from build123d import *

# Parameters (mm, degrees)
SKETCH_1_R             = 2.1
SKETCH_1_R_2           = 1.6
EXTRUDE_1_DEPTH        = 3
HOLE_WIZARD_1_D        = 3.5
HOLE_WIZARD_2_D        = 3.3
PATTERN_LINEAR_1_COUNT = 7
PATTERN_LINEAR_1_PITCH = 15
PATTERN_LINEAR_2_COUNT = 4
PATTERN_LINEAR_2_PITCH = 10
HOLE_WIZARD_3_D        = 3.3
PATTERN_LINEAR_3_COUNT = 7
PATTERN_LINEAR_3_PITCH = 10
HOLE_WIZARD_4_D        = 3.3
SKETCH_14_W            = 20
SKETCH_14_H            = 20
CUT_EXTRUDE_1_DEPTH    = 10
FILLET_1_R             = 3


with BuildPart() as part:
    # 草图1 → 凸台-拉伸1 (new body)
    with BuildSketch(Plane(origin=(0, 0, 0), x_dir=(1, 0, 0), z_dir=(0, 1, 0))):
        with BuildLine():
            Line((-95, 3), (-95, 209))
            ThreePointArc((-95, 209), (-94.121320344, 211.121320344), (-92, 212))
            Line((-92, 212), (92, 212))
            ThreePointArc((92, 212), (94.121320344, 211.121320344), (95, 209))
            Line((95, 209), (95, 3))
            ThreePointArc((95, 3), (94.121320344, 0.878679656), (92, 0))
            Line((92, 0), (56, 0))
            ThreePointArc((56, 0), (53.878679656, 0.878679656), (53, 3))
            Line((53, 3), (53, 43))
            ThreePointArc((53, 43), (44.213203436, 64.213203436), (23, 73))
            Line((23, 73), (-23, 73))
            ThreePointArc((-23, 73), (-44.213203436, 64.213203436), (-53, 43))
            Line((-53, 43), (-53, 3))
            ThreePointArc((-53, 3), (-53.878679656, 0.878679656), (-56, 0))
            Line((-56, 0), (-92, 0))
            ThreePointArc((-92, 0), (-94.121320344, 0.878679656), (-95, 3))
        make_face()
        with Locations(Location((-11.75, 96.75, 0), (0, 0, 270))):
            Circle(SKETCH_1_R, mode=Mode.SUBTRACT)
        with Locations(Location((11.75, 96.75, 0), (0, 0, 270))):
            Circle(SKETCH_1_R, mode=Mode.SUBTRACT)
        with Locations(Location((11.75, 79.25, 0), (0, 0, 270))):
            Circle(SKETCH_1_R, mode=Mode.SUBTRACT)
        with Locations(Location((-11.75, 79.25, 0), (0, 0, 270))):
            Circle(SKETCH_1_R, mode=Mode.SUBTRACT)
        with Locations(Location((-85, 204, 0), (0, 0, 270))):
            Circle(SKETCH_1_R_2, mode=Mode.SUBTRACT)
        with Locations(Location((-61, 204, 0), (0, 0, 270))):
            Circle(SKETCH_1_R_2, mode=Mode.SUBTRACT)
        with Locations(Location((-61, 8, 0), (0, 0, 270))):
            Circle(SKETCH_1_R_2, mode=Mode.SUBTRACT)
        with Locations(Location((-85, 8, 0), (0, 0, 270))):
            Circle(SKETCH_1_R_2, mode=Mode.SUBTRACT)
        with Locations(Location((85, 8, 0), (0, 0, 90))):
            Circle(SKETCH_1_R_2, mode=Mode.SUBTRACT)
        with Locations(Location((61, 8, 0), (0, 0, 90))):
            Circle(SKETCH_1_R_2, mode=Mode.SUBTRACT)
        with Locations(Location((61, 204, 0), (0, 0, 90))):
            Circle(SKETCH_1_R_2, mode=Mode.SUBTRACT)
        with Locations(Location((85, 204, 0), (0, 0, 90))):
            Circle(SKETCH_1_R_2, mode=Mode.SUBTRACT)
        with Locations(Location((85, 64, 0), (0, 0, 270))):
            Circle(SKETCH_1_R_2, mode=Mode.SUBTRACT)
        with Locations(Location((61, 64, 0), (0, 0, 270))):
            Circle(SKETCH_1_R_2, mode=Mode.SUBTRACT)
        with Locations(Location((-85, 64, 0), (0, 0, 90))):
            Circle(SKETCH_1_R_2, mode=Mode.SUBTRACT)
        with Locations(Location((-61, 64, 0), (0, 0, 90))):
            Circle(SKETCH_1_R_2, mode=Mode.SUBTRACT)
        with BuildLine():
            Line((-56, 186), (-56, 162))
            ThreePointArc((-56, 162), (-55.121320344, 159.878679656), (-53, 159))
            Line((-53, 159), (-43, 159))
            ThreePointArc((-43, 159), (-40.878679656, 159.878679656), (-40, 162))
            Line((-40, 162), (-40, 186))
            ThreePointArc((-40, 186), (-40.878679656, 188.121320344), (-43, 189))
            Line((-43, 189), (-53, 189))
            ThreePointArc((-53, 189), (-55.121320344, 188.121320344), (-56, 186))
        make_face(mode=Mode.SUBTRACT)
        with BuildLine():
            Line((43, 189), (53, 189))
            ThreePointArc((53, 189), (55.121320344, 188.121320344), (56, 186))
            Line((56, 186), (56, 162))
            ThreePointArc((56, 162), (55.121320344, 159.878679656), (53, 159))
            Line((53, 159), (43, 159))
            ThreePointArc((43, 159), (40.878679656, 159.878679656), (40, 162))
            Line((40, 162), (40, 186))
            ThreePointArc((40, 186), (40.878679656, 188.121320344), (43, 189))
        make_face(mode=Mode.SUBTRACT)
        with BuildLine():
            Line((77, 139.5), (88, 139.5))
            ThreePointArc((88, 139.5), (89.414213562, 138.914213562), (90, 137.5))
            Line((90, 137.5), (90, 116.5))
            ThreePointArc((90, 116.5), (89.414213562, 115.085786438), (88, 114.5))
            Line((88, 114.5), (77, 114.5))
            ThreePointArc((77, 114.5), (75.585786438, 113.914213562), (75, 112.5))
            Line((75, 112.5), (75, 103))
            ThreePointArc((75, 103), (74.414213562, 101.585786438), (73, 101))
            Line((73, 101), (25, 101))
            ThreePointArc((25, 101), (23.585786438, 101.585786438), (23, 103))
            Line((23, 103), (23, 151))
            ThreePointArc((23, 151), (23.585786438, 152.414213562), (25, 153))
            Line((25, 153), (73, 153))
            ThreePointArc((73, 153), (74.414213562, 152.414213562), (75, 151))
            Line((75, 151), (75, 141.5))
            ThreePointArc((75, 141.5), (75.585786438, 140.085786438), (77, 139.5))
        make_face(mode=Mode.SUBTRACT)
        with BuildLine():
            Line((-14, 166), (14, 166))
            ThreePointArc((14, 166), (16.828427125, 167.171572875), (18, 170))
            Line((18, 170), (18, 198))
            ThreePointArc((18, 198), (16.828427125, 200.828427125), (14, 202))
            Line((14, 202), (-14, 202))
            ThreePointArc((-14, 202), (-16.828427125, 200.828427125), (-18, 198))
            Line((-18, 198), (-18, 170))
            ThreePointArc((-18, 170), (-16.828427125, 167.171572875), (-14, 166))
        make_face(mode=Mode.SUBTRACT)
    extrude(amount=EXTRUDE_1_DEPTH)

    # 孔1 (through all)
    with Locations(Plane(origin=(0, 0, 0), x_dir=(-1, 0, 0), z_dir=(0, -1, 0))):
        with Locations((90, 129.5), (57.5, 129.5), (25, 129.5)):
            Hole(HOLE_WIZARD_1_D / 2)

    # 孔2 (through all)
    with Locations(Plane(origin=(0, 3, 0), x_dir=(1, 0, 0), z_dir=(0, 1, 0))):
        with Locations((13, 142)):
            hole_wizard_2 = Hole(HOLE_WIZARD_2_D / 2)

    # 阵列(线性)1: 孔2 ×7
    with Locations(*[(-i * PATTERN_LINEAR_1_PITCH, 0, 0) for i in range(1, PATTERN_LINEAR_1_COUNT)]):
        add(hole_wizard_2, mode=Mode.SUBTRACT)

    # 阵列(线性)2: 孔2 ×4
    with Locations(*[(0, 0, i * PATTERN_LINEAR_2_PITCH) for i in range(1, PATTERN_LINEAR_2_COUNT)]):
        add(hole_wizard_2, mode=Mode.SUBTRACT)

    # 孔3 (through all)
    with Locations(Plane(origin=(0, 3, 0), x_dir=(1, 0, 0), z_dir=(0, 1, 0))):
        with Locations((25, 90)):
            hole_wizard_3 = Hole(HOLE_WIZARD_3_D / 2)

    # 阵列(线性)3: 孔3 ×7
    with Locations(*[(i * PATTERN_LINEAR_3_PITCH, 0, 0) for i in range(1, PATTERN_LINEAR_3_COUNT)]):
        add(hole_wizard_3, mode=Mode.SUBTRACT)

    # 孔4 (through all)
    with Locations(Plane(origin=(0, 3, 0), x_dir=(1, 0, 0), z_dir=(0, 1, 0))):
        with Locations((85, 105)):
            Hole(HOLE_WIZARD_4_D / 2)

    # 草图14 → 切除-拉伸1 (cut)
    with BuildSketch(Plane(origin=(0, 3, 0), x_dir=(1, 0, 0), z_dir=(0, 1, 0))):
        with Locations((-5, 122)):
            Rectangle(SKETCH_14_W, SKETCH_14_H)
    extrude(amount=-CUT_EXTRUDE_1_DEPTH, mode=Mode.SUBTRACT)

    # 圆角1
    fillet_1_edges = [part.edges().sort_by_distance(p)[0] for p in [
        (-15, 1.5, -112),
        (-15, 1.5, -132),
        (5, 1.5, -132),
        (5, 1.5, -112),
    ]]
    fillet(fillet_1_edges, radius=FILLET_1_R)


solid = part.part
Verification items for the finished model (mm, model axes). A direction names the side the tool comes from. Round coordinates to 2 decimals unless told otherwise and drop trailing zeros. Loops run counter-clockwise (first coordinate to the right, second up) from the corner with the lowest first, then second, coordinate; pieces in that order, holes last. Notation, with made-up numbers: (-38.5, 32) - (2.5, 32) arc R28 cw to (2.5, 59) - close; hole circle Ø1 at (20.5, -12). An arc over 180 degrees is marked (long way). Use a Markdown table: item, result. Add a question column.
1. Gauge pin test, flat end, axial feed: pin 1 (1.5 mm diameter, centred on x = -2, y = 1, fed in from +Z). Record the tip position at first contact, or that the pin passes through.
2. Access from +Z, -Z, +X, -X, +Y, -Y to the whole of each face (thin tool, end or side, straight path). Record for faces 1 (the face through (44.445, 1.479, -63.979)), 2 (the face through (1, 0, -107)).
3. Section check A-A, the plane z = -53.5. Record the boundary of the cut face in (x, y), plus the area to 3 significant figures.
4. Thickness scan on probe 1 along X at (y, z) = (0.2, -118); probe 2 along X at (y, z) = (1, -12.5); probe 3 along X at (y, z) = (1.95, -161.5). Record the ranges inside material, lowest first. Write a range as [from, to].
5. Section check B-B, the plane y = 1.65. Give the number of separate pieces and of enclosed holes in the cut face, plus the area to 3 significant figures.
Checks:
| question | item | result |
|---|---|---|
| 1 | pin 1 | stops at z = -73 |
| 2 | face 1 | +Z, +Y, -Y |
| 2 | face 2 | +Z, -Z, +X, -X, -Y |
| 3 | outline | (-95, 0) - (-51.1, 0) - (-51.1, 3) - (-95, 3) - close; (51.1, 0) - (95, 0) - (95, 3) - (51.1, 3) - close |
| 3 | area | 263 mm^2 |
| 4 | probe 1 | x = [-95, -15], [5, 23], [90, 95] |
| 4 | probe 2 | x = [-95, -53], [53, 95] |
| 4 | probe 3 | x = [-95, -55.96], [-40.04, 40.04], [55.96, 95] |
| 5 | separate pieces | 1 |
| 5 | enclosed holes | 42 |
| 5 | area | 26,900 mm^2 |
